from build123d import *

# Parameters (mm, degrees)
SKETCH1_W               = 15
SKETCH1_H               = 9.5
BOSS_EXTRUDE2_DEPTH     = 5
CUT_EXTRUDE1_DEPTH      = 11.188841936
CUT_EXTRUDE1_DEPTH_BACK = 11.188841936
SKETCH3_R               = 2
SKETCH4_W               = 3
SKETCH4_H               = 5
BOSS_EXTRUDE3_DEPTH     = 5
FILLET1_R               = 2
SKETCH5_W               = 1.5
SKETCH5_H               = 5
BOSS_EXTRUDE4_DEPTH     = 5
SKETCH6_R               = 10.103320079
SKETCH6_R_2             = 8.103320079
BOSS_EXTRUDE5_DEPTH     = 5


with BuildPart() as part:
    # Sketch1 → Boss-Extrude2 (new body)
    with BuildSketch(Plane.XY):
        Rectangle(SKETCH1_W, SKETCH1_H)
    extrude(amount=-BOSS_EXTRUDE2_DEPTH)

    # Sketch3 → Cut-Extrude1 (cut, two sides: drawn at the far end of the back side and taken through both)
    with BuildSketch(Plane.XY.offset(-CUT_EXTRUDE1_DEPTH_BACK)):
        with Locations((2.75, 0)):
            Circle(SKETCH3_R)
    extrude(amount=CUT_EXTRUDE1_DEPTH + CUT_EXTRUDE1_DEPTH_BACK, mode=Mode.SUBTRACT)

    # Sketch4 → Boss-Extrude3 (add)
    with BuildSketch(Plane(origin=(0, 4.75, 0), x_dir=(1, 0, 0), z_dir=(0, 1, 0))):
        with Locations((0, 2.5)):
            Rectangle(SKETCH4_W, SKETCH4_H)
    extrude(amount=BOSS_EXTRUDE3_DEPTH)

    # Fillet1
    fillet1_edges = [part.edges().sort_by_distance(p)[0] for p in [
        (7.5, 0, 0),
        (-7.5, 0, 0),
    ]]
    fillet(fillet1_edges, radius=FILLET1_R)

    # Sketch5 → Boss-Extrude4 (add)
    with BuildSketch(Plane.XY):
        with Locations((0, 12.25)):
            Rectangle(SKETCH5_W, SKETCH5_H)
    extrude(amount=-BOSS_EXTRUDE4_DEPTH)

    # Sketch6 → Boss-Extrude5 (add)
    with BuildSketch(Plane.XY):
        with Locations((0, 14.75)):
            Circle(SKETCH6_R)
        with Locations((0, 14.75)):
            Circle(SKETCH6_R_2, mode=Mode.SUBTRACT)
    extrude(amount=-BOSS_EXTRUDE5_DEPTH)


solid = part.part
The listing builds one solid part. Answer for the finished solid, in the listing's coordinates (mm). A direction names the side the tool comes from. Coordinates: 2 decimals unless noted, no trailing zeros. Write each loop counter-clockwise with the first axis right and the second up, starting at its lowest first coordinate (ties: lowest second). Pieces come first, ordered by that corner, then holes. Notation, with made-up numbers: (78, -24) -> (100, -24) arc R24 cw to (100, -12) -> close; hole circle Ø7 at (74, 56.25). An arc over 180 degrees is marked (long way). One line per question, with ' | ' between items.
1. Section B-B (y = 0) is taken. Determine the outline of the cut face in (x, z).
Verdict:
outline: (-7.5, -5) -> (0.75, -5) -> (0.75, 0) -> (-5.5, 0) arc R2 ccw to (-7.5, -2) -> close; (4.75, -5) -> (7.5, -5) -> (7.5, -2) arc R2 ccw to (5.5, 0) -> (4.75, 0) -> close
2. Section A-A (x = 0) is taken. Determine the outline of the cut face in (y, z), and give its area (4 significant figures).
Verdict:
outline: (-4.75, -5) -> (14.75, -5) -> (14.75, 0) -> (-4.75, 0) -> close; (22.85, -5) -> (24.85, -5) -> (24.85, 0) -> (22.85, 0) -> close | area: 107.5 mm^2
3. For a pull along Y with two mould halves and no side action, classify faces 5 (the flat face through (1.5, 8, -2)), 6 (the flat face through (0, -4.75, -2)), 7 (the cylindrical face through (2.316, -1.952, -2.535)), 8 (the flat face through (0, 7, -5)) as released by +Y, released by -Y, zero draft, split by the parting line, or undercut.
Verdict:
face 5: undercut | face 6: released by -Y | face 7: undercut | face 8: zero draft
4. Straight lines are drawn through the part: line 1 (X direction, y = 14.5, z = -0.55); line 2 (X direction, y = 0, z = -3.3); line 3 (Y direction, x = 0, z = -3.8). For each, find the intervals that lie inside material, in ascending order.
Verdict:
line 1: x = -10.1 to -8.1, -0.75 to 0.75, 8.1 to 10.1 | line 2: x = -7.5 to 0.75, 4.75 to 7.5 | line 3: y = -4.75 to 14.75, 22.85 to 24.85
5. Given pin 1 Ø1.5 at (y, z) = (8.5, -3.5) entering from +X; pin 2 Ø1.5 at (y, z) = (11.5, -3.5) entering from +X; pin 3 Ø6 at (x, y) = (-1.5, 15) entering from +Z; pin 4 Ø3 at (y, z) = (10.5, -2) entering from +X, each flat-ended and moving along its own axis, determine where each tip first touches the part or whether it passes through.
Verdict:
pin 1: stops at x = 8.48 | pin 2: stops at x = 9.79 | pin 3: stops at z = 0 | pin 4: stops at x = 9.72
6. Section D-D (x = 2.75) is taken. Determine the outline of the cut face in (y, z), and give its area (3 significant figures).
Verdict:
outline: (-4.75, -5) -> (-2, -5) -> (-2, 0) -> (-4.75, 0) -> close; (2, -5) -> (4.75, -5) -> (4.75, 0) -> (2, 0) -> close; (5.03, -5) -> (7.13, -5) -> (7.13, 0) -> (5.03, 0) -> close; (22.37, -5) -> (24.47, -5) -> (24.47, 0) -> (22.37, 0) -> close | area: 48.5 mm^2
7. Section C-C (z = -3.4) is taken. State how many separate pieces and enclosed holes the cut face has, and give its area (3 significant figures).
Verdict:
separate pieces: 1 | enclosed holes: 2 | area: 261 mm^2
8. Which of the six approach directions +Z, -Z, +X, -X, +Y, -Y give full straight-line access (tool end or side, diameter ignored) to faces 1 (the flat face through (7.5, 0, -3)), 2 (the cylindrical face through (6.9, 0.07, -0.57)), 3 (the flat face through (-0.75, 12, -2)), 4 (the flat face through (-7.5, 0, -3))?
Verdict:
face 1: +Z, -Z, +X, -Y | face 2: +Z, +X, -Y | face 3: +Z, -Z | face 4: +Z, -Z, -X, -Y
